Input: part model. Units: mm. Frame: model coordinates. Face numbers are marked on the shaded views. A direction names the side the tool comes from. Coordinates: 2 decimals unless noted, no trailing zeros. Order: outer loops, then holes, each group sorted by start corner. A loop starts at its lowest first (then second) coordinate and runs counter-clockwise, first axis right, second up. Notation, with made-up numbers: (-17.5, 83) -> (0.5, 83) arc R21 cw to (0.5, 102) -> close; hole circle Ø8 at (42, -0.5). An arc over 180 degrees is marked (long way). Write each question's results on one line, items separated by ' | '.
```python
from build123d import *

# Parameters (mm, degrees)
SKETCH1_W                = 57
SKETCH1_H                = 62
BOSS_EXTRUDE1_DEPTH      = 6
SKETCH4_W                = 50.6
SKETCH4_H                = 55.6
CUT_EXTRUDE1_DEPTH       = 4
BOSS_EXTRUDE2_DEPTH      = 3
SKETCH6_R                = 0.9
CUT_EXTRUDE2_DEPTH       = 3
BOSS_EXTRUDE3_DEPTH      = 10.5
SKETCH8_R                = 1.25
CUT_EXTRUDE3_DEPTH       = 7.5
CUT_EXTRUDE4_START       = -7.5
SKETCH9_R                = 1.25
CUT_EXTRUDE4_DEPTH       = 7.5
SKETCH10_W               = 57
SKETCH10_H               = 1.4
BOSS_EXTRUDE4_DEPTH      = 22.6
FILLET2_R                = 5
CUT_EXTRUDE8_DEPTH       = 57.79766999
CUT_EXTRUDE8_DEPTH_BACK  = 57.79766999
SKETCH15_W               = 10
SKETCH15_H               = 3.9
SKETCH18_W               = 10
SKETCH18_H               = 5
CUT_EXTRUDE10_DEPTH      = 78.76718663
FILLET3_R                = 2
CUT_EXTRUDE12_DEPTH      = 80.987993526
SKETCH19_R               = 1.15
CUT_EXTRUDE11_DEPTH      = 79.86301615
SKETCH21_W               = 7.2
SKETCH21_H               = 3
CUT_EXTRUDE13_DEPTH      = 57.79766999
CUT_EXTRUDE14_DEPTH      = 58.761365256
CUT_EXTRUDE14_DEPTH_BACK = 0.6
SKETCH22_W               = 57.4
SKETCH22_H               = 62
BOSS_EXTRUDE6_DEPTH      = 17.6
SKETCH24_W               = 4
SKETCH24_H               = 14
CUT_EXTRUDE15_DEPTH      = 6
SKETCH25_W               = 25
SKETCH25_H               = 2
BOSS_EXTRUDE7_DEPTH      = 2


with BuildPart() as part:
    # Sketch1 → Boss-Extrude1 (new body)
    with BuildSketch(Plane(origin=(0, 0, 0), x_dir=(1, 0, 0), z_dir=(0, 1, 0))):
        Rectangle(SKETCH1_W, SKETCH1_H)
    extrude(amount=BOSS_EXTRUDE1_DEPTH)

    # Sketch4 → Cut-Extrude1 (cut)
    with BuildSketch(Plane(origin=(0, 6, 0), x_dir=(1, 0, 0), z_dir=(0, 1, 0))):
        with Locations((-0.8, 0.8)):
            Rectangle(SKETCH4_W, SKETCH4_H)
    extrude(amount=-CUT_EXTRUDE1_DEPTH, mode=Mode.SUBTRACT)

    # Sketch5 → Boss-Extrude2 (add)
    with BuildSketch(Plane(origin=(0, 2, 0), x_dir=(1, 0, 0), z_dir=(0, 1, 0))):
        with BuildLine():
            Line((-26.1, -27), (-18.1, -27))
            Line((-18.1, -27), (24.5, -27))
            Line((24.5, -27), (24.5, -23.5))
            Line((24.5, -23.5), (-18.1, -23.5))
            ThreePointArc((-18.1, -23.5), (-18.832233047, -21.732233047), (-20.6, -21))
            Line((-20.6, -21), (-26.1, -21))
            Line((-26.1, -21), (-26.1, -27))
        make_face()
        with BuildLine():
            Line((24.5, 23.6), (5.5, 23.6))
            ThreePointArc((5.5, 23.6), (3, 21.1), (5.5, 18.6))
            Line((5.5, 18.6), (24.5, 18.6))
            Line((24.5, 18.6), (24.5, 23.6))
        make_face()
        with BuildLine():
            Line((-26.1, 24.6), (-26.1, 28.6))
            Line((-26.1, 28.6), (-22.1, 28.6))
            ThreePointArc((-22.1, 28.6), (-23.271572875, 25.771572875), (-26.1, 24.6))
        make_face()
    extrude(amount=BOSS_EXTRUDE2_DEPTH)

    # Sketch6 → Cut-Extrude2 (cut)
    with BuildSketch(Plane(origin=(0, 5, 0), x_dir=(1, 0, 0), z_dir=(0, 1, 0))):
        with Locations(Location((5.5, 21.1, 0), (0, 0, 270))):
            Circle(SKETCH6_R)
        with Locations(Location((-21.1, -24.5, 0), (0, 0, 270))):
            Circle(SKETCH6_R)
    extrude(amount=-CUT_EXTRUDE2_DEPTH, mode=Mode.SUBTRACT)

    # Sketch7 → Boss-Extrude3 (add)
    with BuildSketch(Plane.XY.offset(31)):
        with BuildLine():
            Line((-28.5, 0), (-31.964101615, -2))
            ThreePointArc((-31.964101615, -2), (-38.794228634, -0.169872981), (-36.964101615, 6.660254038))
            Line((-36.964101615, 6.660254038), (-28.5, 10))
            Line((-28.5, 10), (-28.5, 0))
        make_face()
        with BuildLine():
            Line((36.964101615, 6.660254038), (28.5, 10))
            Line((28.5, 10), (28.5, 0))
            Line((28.5, 0), (31.964101615, -2))
            ThreePointArc((31.964101615, -2), (38.794228634, -0.169872981), (36.964101615, 6.660254038))
        make_face()
    boss_extrude3 = extrude(amount=-BOSS_EXTRUDE3_DEPTH)

    # Mirror4: Boss-Extrude3 across plane
    add(boss_extrude3.mirror(Plane.XY))

    # Sketch8 → Cut-Extrude3 (cut)
    with BuildSketch(Plane(origin=(0, 0, 20.5), x_dir=(-1, 0, 0), z_dir=(0, 0, -1))):
        with Locations((34.464101615, 2.330127019)):
            Circle(SKETCH8_R)
        with Locations((-34.464101615, 2.330127019)):
            Circle(SKETCH8_R)
    extrude(amount=-CUT_EXTRUDE3_DEPTH, mode=Mode.SUBTRACT)

    # Sketch9 → Cut-Extrude4 (cut)
    with BuildSketch(Plane.XY.offset(-20.5).offset(CUT_EXTRUDE4_START)):
        with Locations(Location((-34.464101615, 2.330127019, 0), (0, 0, 180))):
            Circle(SKETCH9_R)
        with Locations(Location((34.464101615, 2.330127019, 0), (0, 0, 180))):
            Circle(SKETCH9_R)
    extrude(amount=CUT_EXTRUDE4_DEPTH, mode=Mode.SUBTRACT)

    # Sketch10 → Boss-Extrude4 (add)
    with BuildSketch(Plane(origin=(0, 6, 0), x_dir=(1, 0, 0), z_dir=(0, 1, 0))):
        with Locations((0, 30.3)):
            Rectangle(SKETCH10_W, SKETCH10_H)
        with Locations((0, -30.3)):
            Rectangle(SKETCH10_W, SKETCH10_H)
    extrude(amount=BOSS_EXTRUDE4_DEPTH)

    # Fillet2
    fillet2_edges = [part.edges().sort_by_distance(p)[0] for p in [
        (-28.5, 28.6, -30.3),
        (28.5, 28.6, -30.3),
        (-28.5, 28.6, 30.3),
        (28.5, 28.6, 30.3),
    ]]
    fillet(fillet2_edges, radius=FILLET2_R)

    # Sketch15 → Cut-Extrude8 (cut, two sides: drawn at the far end of the back side and taken through both)
    with BuildSketch(Plane(origin=(0, 2, 0), x_dir=(1, 0, 0), z_dir=(0, 1, 0)).offset(-CUT_EXTRUDE8_DEPTH_BACK)):
        with Locations((22.3, 25.55)):
            Rectangle(SKETCH15_W, SKETCH15_H)
    extrude(amount=CUT_EXTRUDE8_DEPTH + CUT_EXTRUDE8_DEPTH_BACK, mode=Mode.SUBTRACT)

    # Sketch18 → Cut-Extrude10 (cut, through all)
    with BuildSketch(Plane(origin=(0, 0, 29.6), x_dir=(-1, 0, 0), z_dir=(0, 0, -1))):
        with Locations((10.1, 20.7)):
            Rectangle(SKETCH18_W, SKETCH18_H)
    extrude(amount=-CUT_EXTRUDE10_DEPTH, mode=Mode.SUBTRACT)

    # Fillet3
    fillet3_edges = [part.edges().sort_by_distance(p)[0] for p in [
        (-5.1, 18.2, 30.3),
        (-5.1, 23.2, 30.3),
        (-15.1, 23.2, 30.3),
        (-15.1, 18.2, 30.3),
    ]]
    fillet(fillet3_edges, radius=FILLET3_R)

    # Sketch20 → Cut-Extrude12 (cut, through all)
    with BuildSketch(Plane(origin=(-28.5, 0, 0), x_dir=(0, 0, -1), z_dir=(1, 0, 0))):
        with BuildLine():
            Line((29.6, 8), (29.6, 10))
            Line((29.6, 10), (20.5, 10))
            Line((20.5, 10), (20.5, 8))
            Line((20.5, 8), (21.1, 8))
            ThreePointArc((21.1, 8), (22.1, 7), (23.1, 8))
            Line((23.1, 8), (29.6, 8))
        make_face()
    extrude(amount=-CUT_EXTRUDE12_DEPTH, mode=Mode.SUBTRACT)

    # Sketch19 → Cut-Extrude11 (cut, through all)
    with BuildSketch(Plane.XY.offset(31)):
        with Locations((-23.5, 23.6)):
            Circle(SKETCH19_R)
        with Locations((23.5, 23.6)):
            Circle(SKETCH19_R)
    extrude(amount=-CUT_EXTRUDE11_DEPTH, mode=Mode.SUBTRACT)

    # Sketch21 → Cut-Extrude13 (cut, through all)
    with BuildSketch(Plane(origin=(0, 2, 0), x_dir=(1, 0, 0), z_dir=(0, 1, 0))):
        with Locations((20.9, 22.1)):
            Rectangle(SKETCH21_W, SKETCH21_H)
    extrude(amount=-CUT_EXTRUDE13_DEPTH, mode=Mode.SUBTRACT)

    # Sketch22 → Cut-Extrude14 (cut, two sides: drawn at the far end of the back side and taken through both)
    with BuildSketch(Plane.XZ.offset(-CUT_EXTRUDE14_DEPTH_BACK)):
        Rectangle(SKETCH22_W, SKETCH22_H)
    extrude(amount=CUT_EXTRUDE14_DEPTH + CUT_EXTRUDE14_DEPTH_BACK, mode=Mode.SUBTRACT)

    # Sketch23 → Boss-Extrude6 (add)
    with BuildSketch(Plane(origin=(0, 6, 0), x_dir=(1, 0, 0), z_dir=(0, 1, 0))):
        Polygon((24.5, -7.6), (28.5, -7.6), (28.5, 29.6), (27.3, 29.6), (27.3, 14.4), (24.5, 14.4), align=None)
    extrude(amount=BOSS_EXTRUDE6_DEPTH)

    # Sketch24 → Cut-Extrude15 (cut)
    with BuildSketch(Plane(origin=(0, 23.6, 0), x_dir=(1, 0, 0), z_dir=(0, 1, 0))):
        with Locations((26.5, 3.4)):
            Rectangle(SKETCH24_W, SKETCH24_H)
    extrude(amount=-CUT_EXTRUDE15_DEPTH, mode=Mode.SUBTRACT)

    # Sketch25 → Boss-Extrude7 (add)
    with BuildSketch(Plane.XY.offset(-29.6)):
        with Locations((0, 25.6)):
            Rectangle(SKETCH25_W, SKETCH25_H)
    extrude(amount=BOSS_EXTRUDE7_DEPTH)


solid = part.part
```
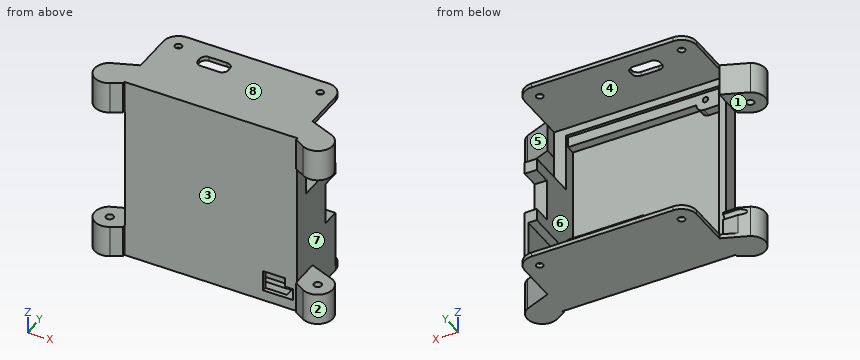
(1) Cut plane B-B, the plane z = 12.5. Return loops of the section in (x, y).
Return value:
outline: (-28.5, 0.6) -> (28.5, 0.6) -> (28.5, 6) -> (24.5, 6) -> (24.5, 2) -> (-26.1, 2) -> (-26.1, 6) -> (-28.5, 6) -> close
(2) Cut plane A-A, the plane y = 13. Return loops of the section in (x, z).
Return value:
outline: (-28.5, -31) -> (28.5, -31) -> (28.5, 7.6) -> (24.5, 7.6) -> (24.5, -14.4) -> (27.3, -14.4) -> (27.3, -29.6) -> (-28.5, -29.6) -> close; (-28.5, 29.6) -> (28.5, 29.6) -> (28.5, 31) -> (-28.5, 31) -> close
(3) Reachability of the marked faces 1, 2, 3, 4 and 5 from +Z, -Z, +X, -X, +Y, -Y: full face, straight path, thin tool, end or side. Return the list, or none.
Return value:
face 1: -X, +Y, -Y | face 2: +Z, -Z | face 3: +Z, -Z, -Y | face 4: +Y | face 5: +Z, -Z, +X, +Y
(4) Cut plane C-C, the plane x = 13.5. Return loops of the section in (y, z), plus the area to 3 significant figures.
Return value:
outline: (0.6, -31) -> (28.6, -31) -> (28.6, -29.6) -> (6, -29.6) -> (6, -28.6) -> (2, -28.6) -> (2, -23.6) -> (5, -23.6) -> (5, -18.6) -> (2, -18.6) -> (2, 23.5) -> (5, 23.5) -> (5, 27) -> (6, 27) -> (6, 29.6) -> (28.6, 29.6) -> (28.6, 31) -> (0.6, 31) -> close | area: 201 mm2
(5) Mould query, pull axis X, two halves, no side actions, for the marked faces 6, 7 and 8. Classes: +X half, -X half, draft (parallel to the pull), parting line (faces both ways), or undercut.
Return value:
face 6: undercut | face 7: +X half | face 8: draft
(6) Cut plane D-D, the plane z = -5. Return loops of the section in (x, y), plus the area to 3 significant figures.
Return value:
outline: (-28.5, 0.6) -> (28.5, 0.6) -> (28.5, 17.6) -> (24.5, 17.6) -> (24.5, 2) -> (-26.1, 2) -> (-26.1, 6) -> (-28.5, 6) -> close | area: 152 mm2
(7) Pin query (flat end, axial travel): P1, Ø4.5, axis at y = 3.5, z = 2.5, coming from the +X side; P2, Ø0.7, axis at x = -9, z = 30.5, coming from the -Y side; P3, Ø1.4, axis at x = -23.5, y = 23.6, coming from the +Z side; P4, Ø10, axis at y = 12.5, z = -16, coming from the -X side. Return the tip coordinate at first contact, or that it passes through.
Return value:
P1: x = 28.5 | P2: y = 0.6 | P3: through | P4: x = 24.5
(8) Line query: line 1 along Z through (x, y) = (6.5, 11); line 2 along X through (y, z) = (4, 17.5); line 3 along X through (y, z) = (23, 30). Output: solid intervals per line, ascending. Write a range as from..to.
Return value:
line 1: -31..-29.6, 29.6..31 | line 2: -28.5..-26.1, 24.5..28.5 | line 3: -28.5..-24.48, -22.52..-13.97, -6.23..22.52, 24.48..28.5
